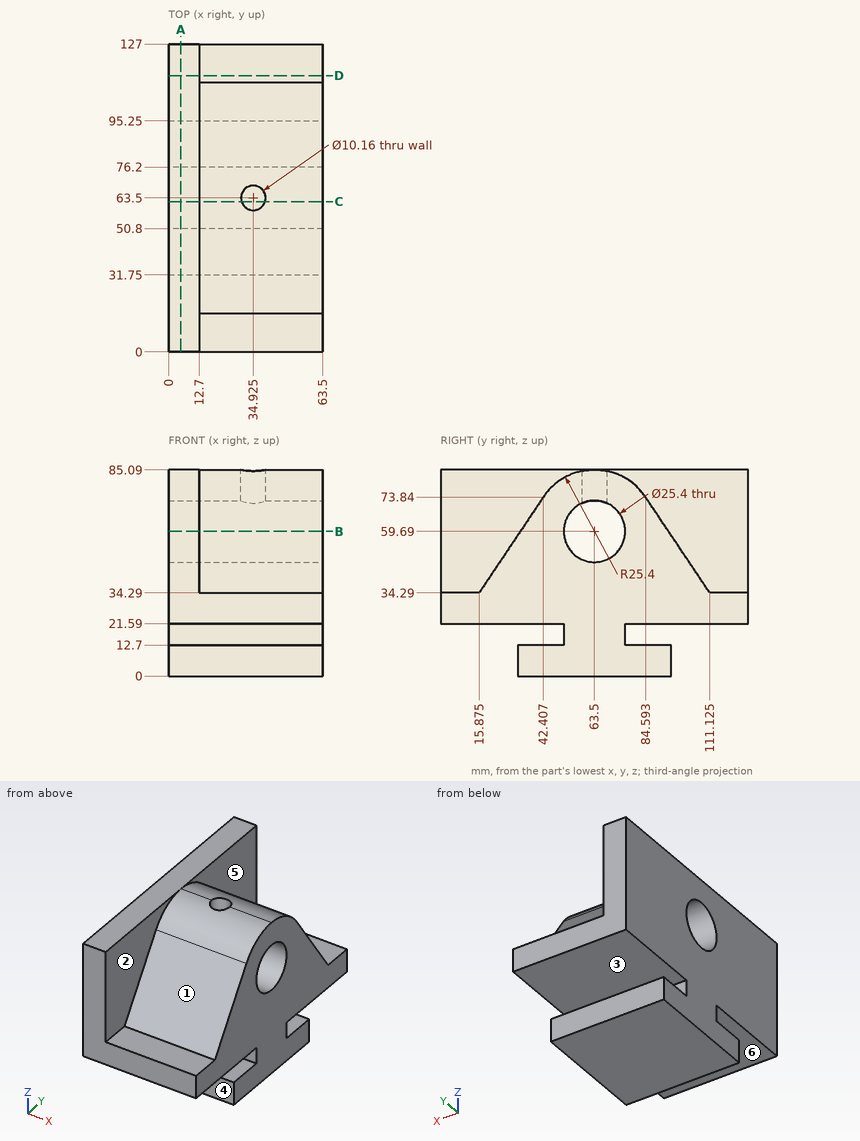
The drawing under review shows one solid part. Ordinate dimensions are in mm from its lowest x, y, z. A direction names the side the tool comes from. Give positions to 0.01 mm unless a question says otherwise; leave off trailing zeros. Order: outer loops, then holes, each group sorted by start corner. A loop starts at its lowest first (then second) coordinate and runs counter-clockwise, first axis right, second up. Notation, with made-up numbers: (19, 10) - (66, 10) arc R14 cw to (66, 14) - close; hole circle Ø3 at (-13, 11). An arc over 180 degrees is marked (long way). Answer as a JSON object with one key per item and string values. Group by question number.
Item 1: Draft analysis for pull direction Z (two halves, no side actions). For the marked faces 1, 2 and 3, state which applies: pulls with the +Z half, pulls with the -Z half, needs draft (parallel to the pull), parting line crosses it, or undercut.
Item 2: Wall thickness on line 1 along Z through (x, y) = (21.5, 63.5); line 2 along Z through (x, y) = (49.5, 14); line 3 along X through (y, z) = (34.5, 65.5): over which ranges is each line inside the solid? List them lowest first.
Item 3: Machinability: for the marked faces 4, 5 and 6, which of the approach directions +Z, -Z, +X, -X, +Y, -Y give a long, thin tool a straight path to every point of the face, cutting with its end or side? Answer none if there is none.
Item 4: Take a section at C-C on y = 62. Give the number of separate pieces and of enclosed holes in the cut face, and give its area (3 significant figures).
Item 5: Take a section at B-B on z = 59.69. Give the boundary of the cut face in (x, y) (1 decimal), and give its area (3 significant figures).
Item 6: Clearance check with flat-ended pins moving along their axes: pin 1 Ø7 at (x, z) = (38, 17.5) entering from +Y; pin 2 Ø6.5 at (x, z) = (42.5, 5) entering from -Y; pin 3 Ø5.5 at (x, y) = (25, 82) entering from +Z. State where each tip first meets the part, or that it passes through.
Item 7: Take a section at A-A on x = 5. Give the boundary of the cut face in (y, z), and give its area (3 significant figures).
Item 8: Take a section at D-D on y = 114. Give the boundary of the cut face in (x, z).
Reported:
{
 "1": {"face 1": "pulls with the +Z half", "face 2": "needs draft", "face 3": "undercut"},
 "2": {"line 1": "0 to 46.99, 72.39 to 85.09", "line 2": "21.59 to 34.29", "line 3": "0 to 12.7"},
 "3": {"face 4": "-Z, +X, -X, -Y", "face 5": "+Z, +X, +Y", "face 6": "+X, -X, -Y"},
 "4": {"separate pieces": "3", "enclosed holes": "0", "area": "3,680 mm^2"},
 "5": {"outline": "(0, 0) - (12.7, 0) - (12.7, 32.9) - (63.5, 32.9) - (63.5, 50.8) - (0, 50.8) - close; (0, 76.2) - (63.5, 76.2) - (63.5, 94.1) - (12.7, 94.1) - (12.7, 127) - (0, 127) - close", "area": "3,110 mm^2"},
 "6": {"pin 1": "y = 76.2", "pin 2": "y = 31.75", "pin 3": "z = 79.62"},
 "7": {"outline": "(0, 21.59) - (50.8, 21.59) - (50.8, 12.7) - (31.75, 12.7) - (31.75, 0) - (95.25, 0) - (95.25, 12.7) - (76.2, 12.7) - (76.2, 21.59) - (127, 21.59) - (127, 85.09) - (0, 85.09) - close; hole circle Ø25.4 at (63.5, 59.69)", "area": "8,590 mm^2"},
 "8": {"outline": "(0, 21.59) - (63.5, 21.59) - (63.5, 34.29) - (12.7, 34.29) - (12.7, 85.09) - (0, 85.09) - close"}
}
